Geometry: final body of the model. Coordinates: model frame, mm. A direction names the side the tool comes from. Round coordinates to 2 decimals unless told otherwise and drop trailing zeros. Loops run counter-clockwise (first coordinate to the right, second up) from the corner with the lowest first, then second, coordinate; pieces in that order, holes last. Notation, with made-up numbers: (81, 47.25) - (122, 47.25) arc R23 cw to (122, 59.25) - close; hole circle Ø8 at (34, 17). An arc over 180 degrees is marked (long way). Return JSON: item names as keys, results as strings. Group by question number.
1. Draft query along Z for faces 1 (the face through (-330, 814, 80)), 2 (the face through (-403.8, 784.2, 37)), 3 (the face through (-534.825, 688.687, 39.44)), 4 (the face through (-267.512, 840.676, 46.085)). Return one class per face: +Z half, -Z half, draft (parallel to the pull), parting line (faces both ways), or undercut.
2. Section A-A on z = 7.5. Return loops of the section in (x, y).
3. First-contact query: pin 1 Ø4 at (x, z) = (-338.5, 48) entering from -Y; pin 2 Ø6 at (x, z) = (-67, 63) entering from -Y; pin 3 Ø1 at (y, z) = (791.5, 47.5) entering from +X. Flat tips, straight axial feed; report the tip coordinate or a pass-through.
4. Set-up query: faces 5 (the face through (-109, 857.154, 39)), 6 (the face through (-109, 865.154, 39)). Return all of +Z, -Z, +X, -X, +Y, -Y with unobstructed straight access to the full face (end or side cutting, diameter ignored); none if empty.
5. Section B-B on x = -176.5. Return loops of the section in (y, z), and give its area (3 significant figures).
6. Material intervals for probe 1 along Y at (x, z) = (-45, 38.5); probe 2 along X at (y, z) = (843.5, 47.5); probe 3 along Y at (x, z) = (-538.5, 23), sorted ascending.
7. Section C-C on y = 725. Return loops of the section in (x, z), and give its area (3 significant figures).
Autodesk Inventor part; units mm, degrees
ref_plane "YZ Plane" through (0, 0, 0) normal (1, 0, 0) x (0, 1, 0)
ref_plane "XZ Plane" through (0, 0, 0) normal (0, 1, 0) x (-1, 0, 0)
ref_plane "XY Plane" through (0, 0, 0) normal (0, 0, 1) x (1, 0, 0)
sketch "Sketch2" plane through (0, 0, 0) normal (0, 0, 1) x (1, 0, 0)
  line L0 (0, 273.8452) -> (193.6378, 193.6378) construction
  line L1 (193.6378, 193.6378) -> (273.8452, 0) construction
  line L2 (273.8452, 0) -> (193.6378, -193.6378) construction
  line L3 (193.6378, -193.6378) -> (0, -273.8452) construction
  line L4 (0, -273.8452) -> (-193.6378, -193.6378) construction
  line L5 (-193.6378, -193.6378) -> (-273.8452, 0) construction
  line L6 (-273.8452, 0) -> (-193.6378, 193.6378) construction
  line L7 (-193.6378, 193.6378) -> (0, 273.8452) construction
  line L8 (-193.6378, 193.6378) -> (0, 273.8452) construction
  line L9 (-459.9272, 770.6562) -> (-219.7185, 870.1539) construction
  line L10 (-96.8189, 233.7415) -> (-339.8229, 820.405) construction
  line L11 (-219.7185, 870.1539) -> (0, 870.1539) construction
  line L12 (0, 870.1539) -> (0, 273.8452) construction
  line L13 (-459.9272, 770.6562) -> (-615.2917, 615.2917) construction
  line L14 (-615.2917, 615.2917) -> (-193.6378, 193.6378) construction
  line L15 (-221.6643, 863.9359) -> (-337.9095, 815.7856)
  line L16 (-5, 865.1539) -> (-215.5414, 865.1539)
  line L17 (-454.1546, 767.6353) -> (-337.9095, 815.7856)
  line L18 (-608.2206, 615.2917) -> (-459.3454, 764.1669)
  arc A0 (-215.5414, 865.1539) -> (-221.6643, 863.9359) centre (-215.5414, 849.1539) ccw
  arc A1 (-454.1546, 767.6353) -> (-459.3454, 764.1669) centre (-448.0317, 752.8532) ccw
  point P0 (0, 0)
  point P1 (0, 0)
  point P2 (0, 0)
  point P3 (-218.724, 865.1539)
  point P4 (-457.095, 766.4174)
  dimension "d0" = 506
  dimension "d1" = 260
  dimension "d2" = 635
  dimension "d6" = 5
  dimension "d10" = 5
  dimension "d14" = 5
  dimension "d15" = 16
contour flange "Contour Flange1" sketch "Sketch2" thickness 8 bend radius 8 width 80 along (0, 0, 1) mid plane no both sides no wall seen from (-110.2707, 865.1539, 0) lies toward (0, -1, 0) curves L16 A0 L15 L17 A1 L18
bend "Bend1"
corner "Corner1"
sketch "Sketch3" plane through (-454.1546, 767.6353, 80) normal (-0.3826834, 0.9238795, 0) x (0.9238795, 0.3826834, 0)
  line L0 (125.8228, 80) -> (125.8228, 0) construction
  line L1 (0, 0) -> (251.6457, 0)
  circle A0 centre (43.3228, 40) radius 10
  circle A1 centre (208.3228, 40) radius 10
  point P0 (125.8228, 40)
  dimension "d27" = 20
  dimension "d28" = 82.5
extrude "Extrusion1" cut sketch "Sketch3" against normal up to surface (8 mm away)
equation "\"d0\" = Барабан_габарит_по_кассетам"
equation "\"d1\" = Кассета_длина_грани"
equation "\"d2\" = Кассета_высота"
equation "\"d10\" = d6"
equation "\"d15\" = BendRadius + Thickness"
equation "\"d16\" = Thickness"
equation "\"d17\" = BendReliefWidth"
equation "\"d18\" = BendReliefDepth"
equation "\"d19\" = MinimumRemnant"
equation "\"d20\" = TransitionRadius"
equation "\"d22\" = BendRadius"
equation "\"d24\" = CornerReliefSize"
equation "\"d25\" = GapSize"
equation "\"d26\" = JacobiRadiusSize"
equation "\"BendRadius\" = Thickness"
equation "\"BendReliefWidth\" = Thickness"
equation "\"BendReliefDepth\" = 0.5 * Thickness"
equation "\"CornerReliefSize\" = 4 * Thickness"
equation "\"MinimumRemnant\" = 2 * Thickness"
equation "\"TransitionRadius\" = BendRadius"
equation "\"JacobiRadiusSize\" = BendRadius"
equation "\"GapSize\" = Thickness"
properties part number "ДМФ 0122 Верхний лист"
Taken from the geometry:
{
 "1": {"face 1": "+Z half", "face 2": "undercut", "face 3": "draft", "face 4": "undercut"},
 "2": {"outline": "(-608.22, 615.29) - (-602.56, 609.63) - (-453.69, 758.51) arc R8 cw to (-451.09, 760.24) - (-334.85, 808.39) - (-218.6, 856.55) arc R8 cw to (-215.54, 857.15) - (-5, 857.15) - (-5, 865.15) - (-215.54, 865.15) arc R16 ccw to (-221.66, 863.94) - (-337.91, 815.79) - (-454.15, 767.64) arc R16 ccw to (-459.35, 764.17) - close"},
 "3": {"pin 1": "y = 806.05", "pin 2": "y = 857.15", "pin 3": "x = -374.43"},
 "4": {"face 5": "+Z, -Z, +X, -Y", "face 6": "+Z, -Z, +X, -X, +Y"},
 "5": {"outline": "(857.15, 0) - (865.15, 0) - (865.15, 80) - (857.15, 80) - close", "area": "640 mm2"},
 "6": {"probe 1": "857.15 to 865.15", "probe 2": "-271 to -267.25, -252.93 to -250.1", "probe 3": "673.7 to 685.01"},
 "7": {"outline": "(-498.51, 0) - (-487.2, 0) - (-487.2, 80) - (-498.51, 80) - close", "area": "905 mm2"}
}
